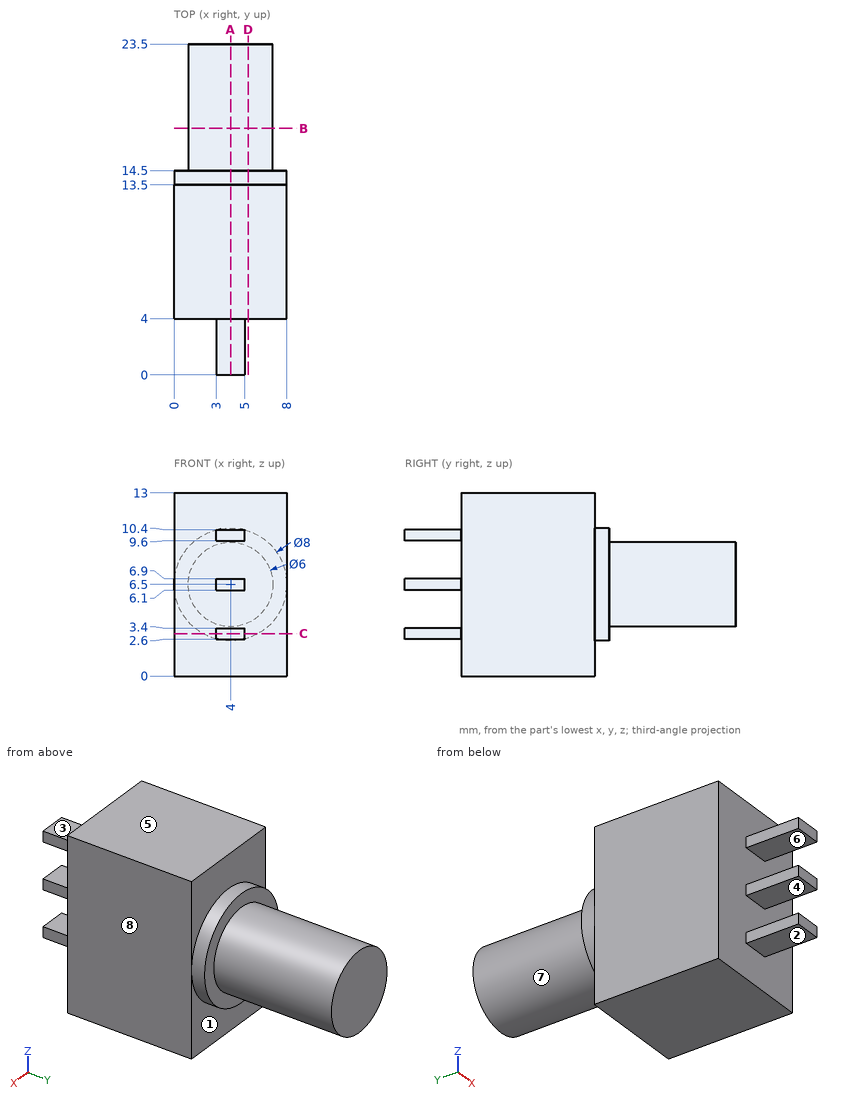
Can you work these out from the drawing? Everything is in mm from the part's minimum corner. A direction names the side the tool comes from. Give positions to 0.01 mm unless a question says otherwise; leave off trailing zeros. Loops run counter-clockwise (first coordinate to the right, second up) from the corner with the lowest first, then second, coordinate; pieces in that order, holes last. Notation, with made-up numbers: (-15.75, 67.25) - (4.25, 67.25) arc R8 cw to (4.25, 75.25) - close; hole circle Ø10 at (-39.75, -0.75). An arc over 180 degrees is marked (long way). Use one line per item in the form item = value.
1. I need wall thicknesses on probe 1 along Y at (x, z) = (6.5, 10.75); probe 2 along Y at (x, z) = (4, 9); probe 3 along X at (y, z) = (19.5, 6). Which ranges of each line are inside material? Lowest first, please.
Response values:
probe_1 = 4 to 13.5
probe_2 = 4 to 23.5
probe_3 = 1.04 to 6.96
2. On a 3-axis mill with a long thin cutter (end or side, diameter ignored), from which of +Z, -Z, +X, -X, +Y, -Y can I reach the whole of each face in a straight line? I mean the marked faces 1, 2, 3 and 4. Say none if no direction works.
Response values:
face_1 = -Z, +Y
face_2 = -Z, +X, -X, -Y
face_3 = +Z, +X, -X, -Y
face_4 = +X, -X, -Y
3. I want a section at C-C (z = 3). Please give me the cut outline in (x, y), and give its area (3 significant figures).
Response values:
outline = (0, 4) - (3, 4) - (3, 0) - (5, 0) - (5, 4) - (8, 4) - (8, 13.5) - (5.94, 13.5) - (5.94, 14.5) - (2.06, 14.5) - (2.06, 13.5) - (0, 13.5) - close
area = 87.9 mm²
4. Thinking about a two-plate mould opening in Z: for the marked faces 5, 6, 7 and 8, which applies, released by +Z, released by -Z, zero draft, split by the parting line, or undercut?
Response values:
face_5 = released by +Z
face_6 = undercut
face_7 = split by the parting line
face_8 = zero draft
5. I want a section at B-B (y = 17.5). Please give me the cut outline in (x, z).
Response values:
outline = circle Ø6 at (4, 6.5)
6. I'm going to push flat-ended pins straight in: pin 1 Ø0.9 at (y, z) = (1, 6.5) entering from -X; pin 2 Ø0.6 at (x, y) = (4.5, 2.5) entering from +Z; pin 3 Ø2 at (x, y) = (4, 2.5) entering from -Z; pin 4 Ø2 at (x, z) = (3.5, 7) entering from -Y. Where does each tip first touch, or does it pass through?
Response values:
pin_1 = 3
pin_2 = 10.4
pin_3 = 2.6
pin_4 = 0
7. I want a section at D-D (x = 5.25). Please give me the cut outline in (y, z).
Response values:
outline = (4, 0) - (13.5, 0) - (13.5, 2.7) - (14.5, 2.7) - (14.5, 3.77) - (23.5, 3.77) - (23.5, 9.23) - (14.5, 9.23) - (14.5, 10.3) - (13.5, 10.3) - (13.5, 13) - (4, 13) - close
8. I want a section at A-A (x = 4). Please give me the cut outline in (y, z).
Response values:
outline = (0, 2.6) - (4, 2.6) - (4, 0) - (13.5, 0) - (13.5, 2.5) - (14.5, 2.5) - (14.5, 3.5) - (23.5, 3.5) - (23.5, 9.5) - (14.5, 9.5) - (14.5, 10.5) - (13.5, 10.5) - (13.5, 13) - (4, 13) - (4, 10.4) - (0, 10.4) - (0, 9.6) - (4, 9.6) - (4, 6.9) - (0, 6.9) - (0, 6.1) - (4, 6.1) - (4, 3.4) - (0, 3.4) - close
